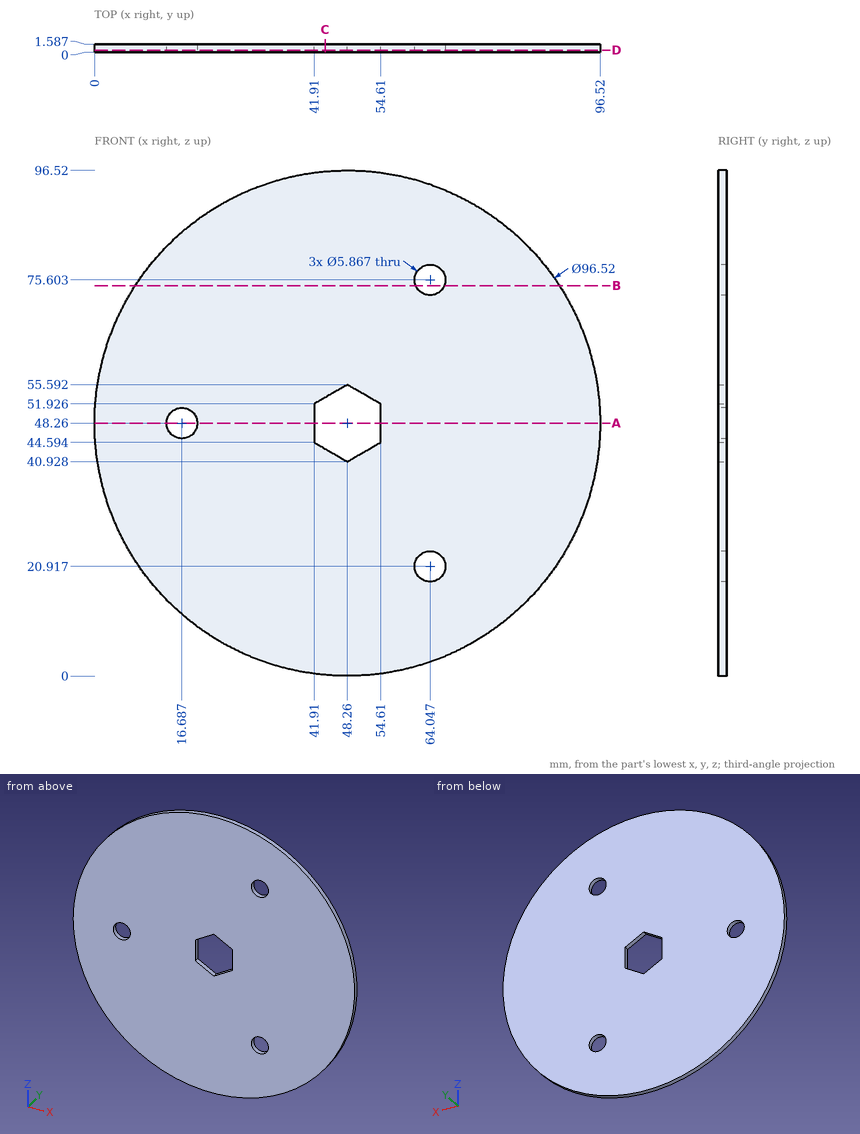
The figure shows three views and two pictorial views of one solid part (mm, origin at its lowest corner). Answer the questions. Coordinates: 2 decimals unless noted, no trailing zeros. Order: outer loops, then holes, each group sorted by start corner. A loop starts at its lowest first (then second) coordinate and runs counter-clockwise, first axis right, second up.
Q1. A cutting plane is placed at C-C, the plane x = 44. Write down the section's boundary in (y, z), and give its area (3 significant figures).
Q2. A cutting plane is placed at B-B, the plane z = 74.5. Write down the section's boundary in (x, y) (1 decimal), and give its area (3 significant figures).
Q3. A cutting plane is placed at A-A, the plane z = 48.26. Write down the section's boundary in (x, y).
Q4. Given P1, Ø3.5, axis at x = 16.69, z = 48.26, coming from the -Y side, flat-ended and moving along its own axis, determine where the tip first touches the part or whether it passes through.
Q5. Consider line 1 (Z direction, x = 62, y = 1.2) (1 decimal); line 2 (Z direction, x = 66, y = 0.8) (1 decimal); line 3 (Z direction, x = 48, y = 1.55). Determine where each line is inside the solid, lowest interval first.
Q6. A cutting plane is placed at D-D, the plane y = 0.4. Write down the section's boundary in (x, z), and give its area (3 significant figures).
Answers follow:
1. outline: (0, 0.19) - (1.59, 0.19) - (1.59, 43.39) - (0, 43.39) - close; (0, 53.13) - (1.59, 53.13) - (1.59, 96.33) - (0, 96.33) - close
1. area: 137 mm2
2. outline: (7.8, 0) - (61.3, 0) - (61.3, 1.6) - (7.8, 1.6) - close; (66.8, 0) - (88.8, 0) - (88.8, 1.6) - (66.8, 1.6) - close
2. area: 120 mm2
3. outline: (0, 0) - (13.75, 0) - (13.75, 1.59) - (0, 1.59) - close; (19.62, 0) - (41.91, 0) - (41.91, 1.59) - (19.62, 1.59) - close; (54.61, 0) - (96.52, 0) - (96.52, 1.59) - (54.61, 1.59) - close
4. P1: passes through
5. line 1: z = 2 to 18.8, 23 to 73.5, 77.7 to 94.5
5. line 2: z = 3.4 to 18.7, 23.1 to 73.4, 77.8 to 93.1
5. line 3: z = 0 to 41.08, 55.44 to 96.52
6. outline: circle Ø96.52 at (48.26, 48.26); hole circle Ø5.87 at (16.69, 48.26); hole (41.91, 44.59) - (48.26, 40.93) - (54.61, 44.59) - (54.61, 51.93) - (48.26, 55.59) - (41.91, 51.93) - close; hole circle Ø5.87 at (64.05, 20.92); hole circle Ø5.87 at (64.05, 75.6)
6. area: 7,100 mm2
